Source: CAD feature listing. Evaluate the final solid. Frame: model axes, mm. Face numbers are marked on the shaded views. A direction names the side the tool comes from. Give positions to 0.01 mm unless a question says otherwise; leave off trailing zeros. Loops run counter-clockwise (first coordinate to the right, second up) from the corner with the lowest first, then second, coordinate; pieces in that order, holes last. Notation, with made-up numbers: M 27,14 L 60,14 A6 cw 60,24 Z; hole C 29,-32.75 d9. An arc over 180 degrees is marked long. Write item = value, one per line.
from build123d import *

# Parameters (mm, degrees)
EXTRUDE_1_DEPTH     = 26
SKETCH_2_R          = 4.75
EXTRUDE_2_DEPTH     = 3
SKETCH_3_R          = 1
EXTRUDE_3_DEPTH     = 4
SKETCH_4_R          = 4.375
T20X0_4_DEPTH       = 2
CUT_EXTRUDE_1_DEPTH = 3
SKETCH_6_R          = 3.135
EXTRUDE_5_DEPTH     = 2.5
SKETCH_7_R          = 1.25
CUT_EXTRUDE_2_DEPTH = 1
SKETCH_8_W          = 1.8
SKETCH_8_H          = 15.2
CUT_EXTRUDE_3_DEPTH = 8


with BuildPart() as part:
    # 草图1 → 凸台-拉伸1 (new body)
    with BuildSketch(Plane.XY):
        with BuildLine():
            Line((-8.294727241, 7.6), (8.294727241, 7.6))
            ThreePointArc((8.294727241, 7.6), (11.25, 0), (8.294727241, -7.6))
            Line((8.294727241, -7.6), (-8.294727241, -7.6))
            ThreePointArc((-8.294727241, -7.6), (-11.25, 0), (-8.294727241, 7.6))
        make_face()
    extrude(amount=EXTRUDE_1_DEPTH)

    # 草图2 → 凸台-拉伸2 (add)
    with BuildSketch(Plane.XY.offset(26)):
        Circle(SKETCH_2_R)
    extrude(amount=EXTRUDE_2_DEPTH)

    # 草图3 → 凸台-拉伸3 (add)
    with BuildSketch(Plane.XY.offset(29)):
        Circle(SKETCH_3_R)
    extrude(amount=EXTRUDE_3_DEPTH)

    # 草图4 → T20x0.4 (add)
    with BuildSketch(Plane.XY.offset(31.4)):
        Circle(SKETCH_4_R)
    extrude(amount=-T20X0_4_DEPTH)

    # 草图5 → 切除-拉伸1 (cut)
    with BuildSketch(Plane(origin=(0, 0, 0), x_dir=(-1, 0, 0), z_dir=(0, 0, -1))):
        with BuildLine():
            Line((8.294727241, -7.6), (-8.294727241, -7.6))
            ThreePointArc((-8.294727241, -7.6), (-11.25, 0), (-8.294727241, 7.6))
            Line((-8.294727241, 7.6), (8.294727241, 7.6))
            ThreePointArc((8.294727241, 7.6), (11.25, 0), (8.294727241, -7.6))
        make_face()
        with BuildLine():
            Line((8.250606038, 7.5), (-8.250606038, 7.5))
            ThreePointArc((-8.250606038, 7.5), (-11.15, 0), (-8.250606038, -7.5))
            Line((-8.250606038, -7.5), (8.250606038, -7.5))
            ThreePointArc((8.250606038, -7.5), (11.15, 0), (8.250606038, 7.5))
        make_face(mode=Mode.SUBTRACT)
    extrude(amount=-CUT_EXTRUDE_1_DEPTH, mode=Mode.SUBTRACT)

    # 草图6 → 凸台-拉伸5 (add)
    with BuildSketch(Plane(origin=(0, 0, 0), x_dir=(-1, 0, 0), z_dir=(0, 0, -1))):
        Circle(SKETCH_6_R)
    extrude(amount=EXTRUDE_5_DEPTH)

    # 草图7 → 切除-拉伸2 (cut)
    with BuildSketch(Plane(origin=(0, 0, -2.5), x_dir=(-1, 0, 0), z_dir=(0, 0, -1))):
        Circle(SKETCH_7_R)
    extrude(amount=-CUT_EXTRUDE_2_DEPTH, mode=Mode.SUBTRACT)

    # 草图8 → 切除-拉伸3 (cut)
    with BuildSketch(Plane(origin=(0, 0, 0), x_dir=(-1, 0, 0), z_dir=(0, 0, -1))):
        with Locations((-10.35, 0)):
            Rectangle(SKETCH_8_W, SKETCH_8_H)
    extrude(amount=-CUT_EXTRUDE_3_DEPTH, mode=Mode.SUBTRACT)


solid = part.part
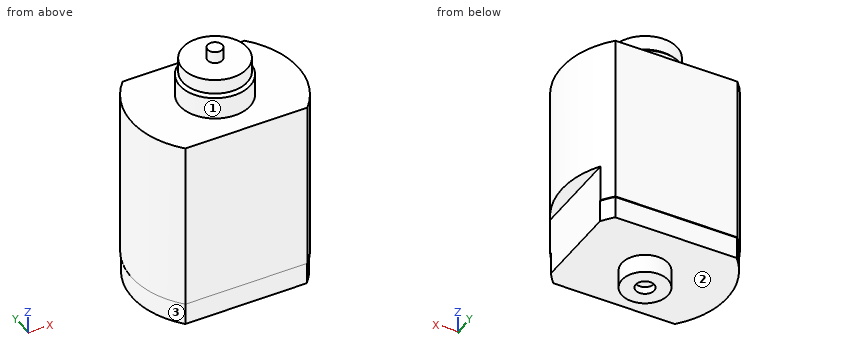
1. Reachability of the marked faces 1, 2 and 3 from +Z, -Z, +X, -X, +Y, -Y: full face, straight path, thin tool, end or side. Return the list, or none.
Derived:
face_1 = +Z
face_2 = -Z
face_3 = -Z, -X
2. Material intervals for probe 1 along Y at (x, z) = (0, -2.3) (3 decimals); probe 2 along Z at (x, y) = (-3, 1.75); probe 3 along Z at (x, y) = (8.5, 1), sorted ascending. Write a range as from..to.
Derived:
probe_1 = -3.135..-1.25, 1.25..3.135
probe_2 = 0..29, 29.4..31.4
probe_3 = 0..26
3. Cut plane C-C, the plane x = 2.25. Return the cut outline in (y, z), then the cut area to 3 significant figures.
Derived:
outline = M -7.6,3 L -7.5,3 L -7.5,0 L -2.18,0 L -2.18,-2.5 L 2.18,-2.5 L 2.18,0 L 7.5,0 L 7.5,3 L 7.6,3 L 7.6,26 L 4.18,26 L 4.18,29 L -4.18,29 L -4.18,26 L -7.6,26 Z; M -3.75,29.4 L 3.75,29.4 L 3.75,31.4 L -3.75,31.4 Z
area = 446 mm²
4. First-contact query: pin 1 Ø6.5 at (y, z) = (1.5, 2) entering from +X; pin 2 Ø2.5 at (x, z) = (1.5, 1.5) entering from +Y; pin 3 Ø0.5 at (x, y) = (10, 2.5) entering from -Z. Flat tips, straight axial feed; report the tip coordinate or a pass-through.
Derived:
pin_1 = 9.45
pin_2 = 7.5
pin_3 = 8
5. Cut plane D-D, the plane z = 6. Return the cut outline in (x, y).
Derived:
outline = M -8.29,-7.6 L 8.29,-7.6 A11.25 ccw 9.45,-6.1 L 9.45,6.1 A11.25 ccw 8.29,7.6 L -8.29,7.6 A11.25 ccw Z
